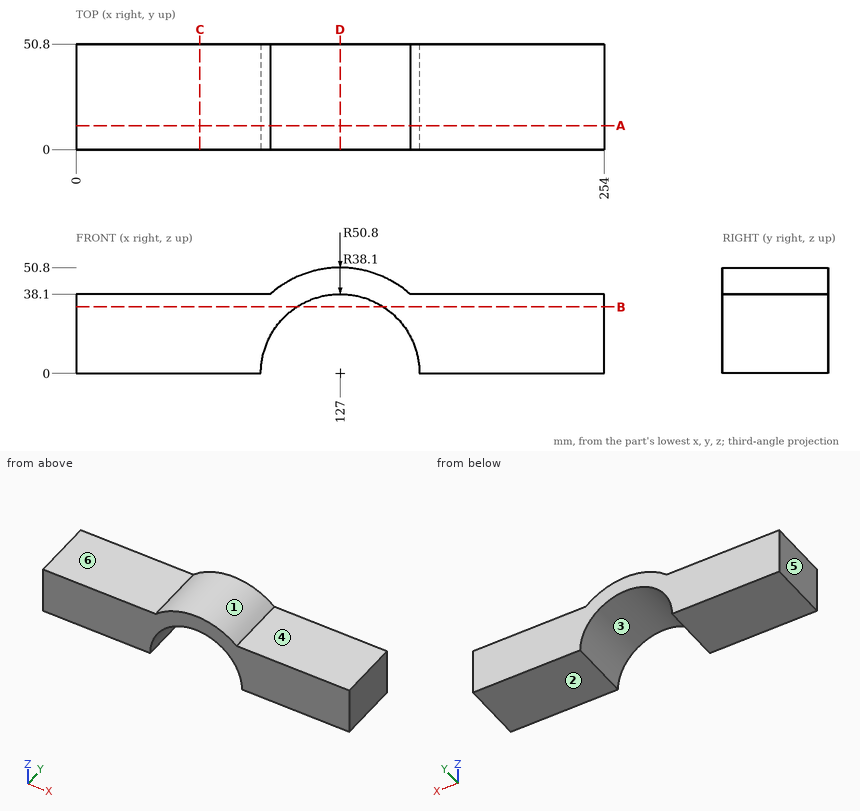
Geometry check sheet. Reference: drawing and pictorial views, mm from the part's lowest x, y, z. A direction names the side the tool comes from. Give positions to 0.01 mm unless a question says otherwise; leave off trailing zeros. Order: outer loops, then holes, each group sorted by start corner. A loop starts at its lowest first (then second) coordinate and runs counter-clockwise, first axis right, second up. Notation, with made-up numbers: M 18,42.5 L 32,42.5 A20 ccw 32,50.5 Z; hole C 6,32 d11. An arc over 180 degrees is marked long. Answer in a Markdown table with one row per item. Add a question column.
Item 1: Tool access check on the marked faces 4, 5 and 6. Record the directions out of +Z, -Z, +X, -X, +Y, -Y that give a thin tool (end or side, any length) a straight path to the whole face; none if there is none.
Item 2: Mould release check, pull along X, two halves, no side actions. Record for the marked faces 1, 2 and 3: released by +X, released by -X, zero draft, split by the parting line, or undercut.
Item 3: Section check D-D, the plane x = 127. Enter the section's corners in (y, z), and give its area (3 significant figures).
Item 4: Section check A-A, the plane y = 11.5. Enter the section's corners in (x, z).
Item 5: Section check C-C, the plane x = 59.5. Enter the section's corners in (y, z), and give its area (3 significant figures).
Item 6: Scan lines: probe 1 along X at (y, z) = (20, 18); probe 2 along Z at (x, y) = (86.5, 42.5); probe 3 along X at (y, z) = (24, 3). Record each from-to range of solid material in increasing order. Write a range as from..to.
Item 7: Gauge pin test, flat ends, axial feed: pin 1 (1.5 mm diameter, centred on x = 162, z = 40.5, fed in from +Y); pin 2 (5 mm diameter, centred on y = 19, z = 17, fed in from -X); pin 3 (8 mm diameter, centred on x = 188.5, y = 28, fed in from +Z). Record the tip position at first contact, or that the pin passes through.
Item 8: Section check B-B, the plane z = 32. Enter the section's corners in (x, y), and give its area (3 significant figures).
Filled sheet:
| question | item | result |
|---|---|---|
| 1 | face 4 | +Z, +X, +Y, -Y |
| 1 | face 5 | +Z, -Z, -X, +Y, -Y |
| 1 | face 6 | +Z, -X, +Y, -Y |
| 2 | face 1 | split by the parting line |
| 2 | face 2 | zero draft |
| 2 | face 3 | undercut |
| 3 | outline | M 0,38.1 L 50.8,38.1 L 50.8,50.8 L 0,50.8 Z |
| 3 | area | 645 mm^2 |
| 4 | outline | M 0,0 L 88.9,0 A38.1 cw 165.1,0 L 254,0 L 254,38.1 L 160.6,38.1 A50.8 ccw 93.4,38.1 L 0,38.1 Z |
| 5 | outline | M 0,0 L 50.8,0 L 50.8,38.1 L 0,38.1 Z |
| 5 | area | 1,940 mm^2 |
| 6 | probe 1 | x = 0..93.42, 160.58..254 |
| 6 | probe 2 | z = 0..38.1 |
| 6 | probe 3 | x = 0..89.02, 164.98..254 |
| 7 | pin 1 | passes through |
| 7 | pin 2 | stops at x = 0 |
| 7 | pin 3 | stops at z = 38.1 |
| 8 | outline | M 0,0 L 106.32,0 L 106.32,50.8 L 0,50.8 Z; M 147.68,0 L 254,0 L 254,50.8 L 147.68,50.8 Z |
| 8 | area | 10,800 mm^2 |
